```python
from build123d import *

# Parameters (mm, degrees)
SKETCH2_R          = 1.5
CUT_EXTRUDE1_DEPTH = 90.582364336
SKETCH3_R          = 20
CUT_EXTRUDE2_DEPTH = 92.454906921


with BuildPart() as part:
    # Sketch1 → Revolve1 (revolve)
    with BuildSketch(Plane.XY, mode=Mode.PRIVATE) as revolve1_sk:
        Polygon((0, 58), (44, 58), (44, 3), (50, 3), (50, 0), (41.5, 0), (41.5, 55), (0, 55), align=None)
    revolve(revolve1_sk.sketch.rotate(Axis((0, 0, 0), (0, 1, 0)), 90), axis=Axis((0, 0, 0), (0, 1, 0)))

    # Sketch2 → Cut-Extrude1 (cut, through all)
    with BuildSketch(Plane(origin=(0, 3, 0), x_dir=(1, 0, 0), z_dir=(0, 1, 0))):
        with Locations(Location((0, -47, 0), (0, 0, 270))):
            Circle(SKETCH2_R)
        with Locations(Location((-33.234018716, -33.234018716, 0), (0, 0, 270))):
            Circle(SKETCH2_R)
        with Locations(Location((-47, 0, 0), (0, 0, 270))):
            Circle(SKETCH2_R)
        with Locations(Location((-33.234018716, 33.234018716, 0), (0, 0, 270))):
            Circle(SKETCH2_R)
        with Locations(Location((0, 47, 0), (0, 0, 270))):
            Circle(SKETCH2_R)
        with Locations(Location((33.234018716, 33.234018716, 0), (0, 0, 270))):
            Circle(SKETCH2_R)
        with Locations(Location((47, 0, 0), (0, 0, 270))):
            Circle(SKETCH2_R)
        with Locations(Location((33.234018716, -33.234018716, 0), (0, 0, 270))):
            Circle(SKETCH2_R)
    extrude(amount=-CUT_EXTRUDE1_DEPTH, mode=Mode.SUBTRACT)

    # Sketch3 → Cut-Extrude2 (cut, through all)
    with BuildSketch(Plane(origin=(0, 58, 0), x_dir=(1, 0, 0), z_dir=(0, 1, 0))):
        with Locations(Location((0, 0, 0), (0, 0, 270))):
            Circle(SKETCH3_R)
    extrude(amount=-CUT_EXTRUDE2_DEPTH, mode=Mode.SUBTRACT)


solid = part.part
```
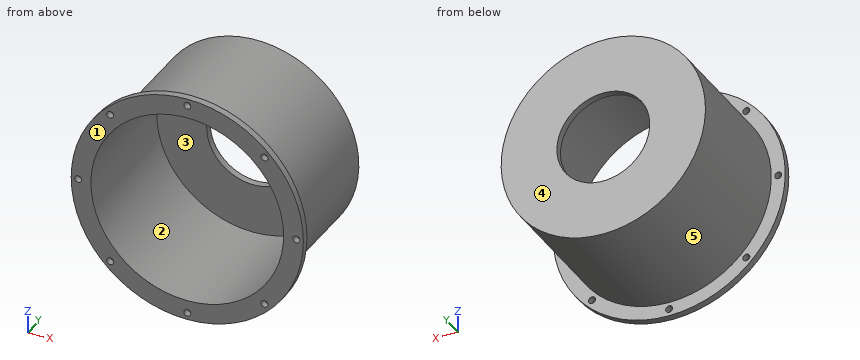
Input: part model. Units: mm. Frame: model coordinates. Face numbers are marked on the shaded views. A direction names the side the tool comes from. Give positions to 0.01 mm unless a question says otherwise; leave off trailing zeros. Write each loop counter-clockwise with the first axis right and the second up, starting at its lowest first coordinate (ties: lowest second). Pieces come first, ordered by that corner, then holes. Notation, with made-up numbers: (19, 11) - (67, 11) arc R19 ccw to (67, 22) - close; hole circle Ø10 at (16.25, -37). An arc over 180 degrees is marked (long way). Write item = value, one per line. Start each with the question number.
1) Reachability of the marked faces 1 and 2 from +Z, -Z, +X, -X, +Y, -Y: full face, straight path, thin tool, end or side. Return the list, or none.
2) Pin query (flat end, axial travel): pin 1 (3.5 mm diameter, centred on x = 0, z = -47, fed in from +Y); pin 2 (3 mm diameter, centred on x = -9, y = 42.5, fed in from -Z); pin 3 (1 mm diameter, centred on x = 39.5, y = 7, fed in from +Z); pin 4 (2.5 mm diameter, centred on x = -33.23, z = 33.23, fed in from +Y). Return the tip coordinate at first contact, or that it passes through.
3) Draft query along Z for the marked faces 3, 4 and 5. Return one class per face: pulls with the +Z half, pulls with the -Z half, needs draft (parallel to the pull), parting line crosses it, or undercut.
4) Cut plane A-A (z = 0). Return loops of the section in (x, y).
5) Cut plane D-D (y = 48). Return loops of the section in (x, z).
6) Cut plane C-C (x = 23.5). Return loops of the section in (y, z).
7) Material intervals for L1, parallel to X at y = 2, z = 0; L2, parallel to Y at x = -8, z = 22; L3, parallel to Y at x = 39.5, z = 22.5, sorted ascending. Write a range as [from, to].
8) Cut plane B-B (z = 47). Return loops of the section in (x, y), and give its area (3 significant figures).
Answers follow:
q1.face_1 = +Z, -Z, +X, -X, -Y
q1.face_2 = -Y
q2.pin_1 = 3
q2.pin_2 = -43.36
q2.pin_3 = 20.37
q2.pin_4 = through
q3.face_3 = undercut
q3.face_4 = needs draft
q3.face_5 = parting line crosses it
q4.outline = (-50, 0) - (-48.5, 0) - (-48.5, 3) - (-50, 3) - close; (-45.5, 0) - (-41.5, 0) - (-41.5, 55) - (-20, 55) - (-20, 58) - (-44, 58) - (-44, 3) - (-45.5, 3) - close; (20, 55) - (41.5, 55) - (41.5, 0) - (45.5, 0) - (45.5, 3) - (44, 3) - (44, 58) - (20, 58) - close; (48.5, 0) - (50, 0) - (50, 3) - (48.5, 3) - close
q5.outline = circle Ø88 at (0, 0); hole circle Ø83 at (0, 0)
q6.outline = (0, -44.13) - (3, -44.13) - (3, -37.2) - (58, -37.2) - (58, 37.2) - (3, 37.2) - (3, 44.13) - (0, 44.13) - (0, 34.21) - (55, 34.21) - (55, -34.21) - (0, -34.21) - close
q7.L1 = [-50, -48.5], [-45.5, -41.5], [41.5, 45.5], [48.5, 50]
q7.L2 = [55, 58]
q7.L3 = [0, 3]
q8.outline = (-17.06, 0) - (-1.5, 0) - (-1.5, 3) - (-17.06, 3) - close; (1.5, 0) - (17.06, 0) - (17.06, 3) - (1.5, 3) - close
q8.area = 93.4 mm^2
